Can you work these out from the model? Positions are in its coordinate system, mm. A direction names the side the tool comes from. Coordinates: 2 decimals unless noted, no trailing zeros. Loops run counter-clockwise (first coordinate to the right, second up) from the corner with the lowest first, then second, coordinate; pieces in that order, holes last. Notation, with made-up numbers: M -3.75,70.5 L 37.25,70.5 A26 cw 37.25,86.5 Z; hole C 22,85.5 d4. An arc over 180 degrees is marked long. Answer as a JSON object with one key per item and string values. Group by question number.
Item 1: Suppose I cut it at A-A (y = 0). Write out the boundary of the cut face in (x, z).
Item 2: Suppose I cut it at B-B (x = 0). Write out the boundary of the cut face in (y, z).
Item 3: I'm going to push a flat-ended pin straight in: pin 1 Ø5.5 at (x, y) = (1.5, 1.5) entering from -Z. Where does the tip first touch, or does it pass through?
Item 4: Which directions (+Z, -Z, +X, -X, +Y, -Y) give clear straight access to the entire face, cutting with the end or side of a thin tool? Please do faces 4 (the flat face through (-6, 0, -114.3)), 5 (the flat face through (0, 0, -83.058)).
Item 5: We'd pull the mould along Y, two halves only. Please class faces 1 (the cylindrical face through (2.472, -4.754, -98.46)), 2 (the flat face through (12.7, 0, 2)), 3 (the flat face through (0, 7.938, 2)): +Y half, -Y half, draft (parallel to the pull), parting line (faces both ways), or undercut.
Item 6: If I drill on line 1 (Y direction, x = 0, z = -92); line 2 (Z direction, x = 2.5, y = 2.25); line 3 (Y direction, x = 1.5, z = -92), over which ranges is the centre line in solid material (lowest first)?
```python
from build123d import *

# Parameters (mm, degrees)
SKETCH1_W                   = 25.4
SKETCH1_H                   = 15.875
BOSS_EXTRUDE1_DEPTH         = 114.3
F_1_2_13_TAPPED_HOLE1_D     = 10.71626
F_1_2_13_TAPPED_HOLE1_DEPTH = 31.242


with BuildPart() as part:
    # Sketch1 → Boss-Extrude1 (new body, symmetric)
    with BuildSketch(Plane.XY):
        Rectangle(SKETCH1_W, SKETCH1_H)
    extrude(amount=BOSS_EXTRUDE1_DEPTH, both=True)

    # 1/2-13 Tapped Hole1
    with Locations(Plane(origin=(0, 0, -114.3), x_dir=(-1, 0, 0), z_dir=(0, 0, -1))):
        with Locations((0, 0)):
            Hole(F_1_2_13_TAPPED_HOLE1_D / 2, depth=F_1_2_13_TAPPED_HOLE1_DEPTH)


solid = part.part
```
From the geometry:
{
 "1": {"outline": "M -12.7,-114.3 L -5.36,-114.3 L -5.36,-83.06 L 5.36,-83.06 L 5.36,-114.3 L 12.7,-114.3 L 12.7,114.3 L -12.7,114.3 Z"},
 "2": {"outline": "M -7.94,-114.3 L -5.36,-114.3 L -5.36,-83.06 L 5.36,-83.06 L 5.36,-114.3 L 7.94,-114.3 L 7.94,114.3 L -7.94,114.3 Z"},
 "3": {"pin 1": "z = -83.06"},
 "4": {"face 4": "-Z, +X, -X, +Y, -Y", "face 5": "-Z"},
 "5": {"face 1": "undercut", "face 2": "draft", "face 3": "+Y half"},
 "6": {"line 1": "-7.94 to -5.36, 5.36 to 7.94", "line 2": "-83.06 to 114.3", "line 3": "-7.94 to -5.14, 5.14 to 7.94"}
}
